Source: CAD feature listing. Evaluate the final solid. Frame: model axes, mm. A direction names the side the tool comes from. Give positions to 0.01 mm unless a question says otherwise; leave off trailing zeros. Write each loop counter-clockwise with the first axis right and the second up, starting at its lowest first coordinate (ties: lowest second). Pieces come first, ordered by that corner, then holes. Notation, with made-up numbers: (49, -2.5) -> (70, -2.5) arc R31 ccw to (70, 32.5) -> close; hole circle Ø8 at (43, -34). An arc over 180 degrees is marked (long way). Write item = value, one per line.
Autodesk Inventor part; units mm, degrees
ref_plane "YZ Plane" through (0, 0, 0) normal (1, 0, 0) x (0, 1, 0)
ref_plane "XZ Plane" through (0, 0, 0) normal (0, 1, 0) x (-1, 0, 0)
ref_plane "XY Plane" through (0, 0, 0) normal (0, 0, 1) x (1, 0, 0)
sketch "Skizze1" plane through (0, 0, 0) normal (0, 0, 1) x (1, 0, 0)
  line L0 (-60, 110) -> (60, 110)
  line L1 (60, 110) -> (60, -10)
  line L2 (60, -10) -> (-60, -10)
  line L3 (-60, -10) -> (-60, 110)
  point P0 (0, 0)
  point P1 (0, 110)
  dimension "d0" = 120
  dimension "d1" = 120
  dimension "d2" = 10
extrude "Extrusion1" add sketch "Skizze1" against normal blind 5
sketch "Skizze2" plane through (0, 0, 0) normal (0, 0, 1) x (1, 0, 0)
  line L0 (-60, -10) -> (-60, 110)
  line L1 (-60, 0) -> (-10.5, 0)
  line L2 (-10.5, 0) -> (-10.5, 110)
  line L3 (-60, 110) -> (60, 110)
  line L4 (-5, 110) -> (-5, 0)
  line L5 (-5, 0) -> (60, 0)
  line L6 (-60, -10) -> (60, -10)
  line L7 (60, -10) -> (-60, -10)
  line L8 (60, 110) -> (60, -10)
  line L9 (-10.5, 110) -> (-5, 110)
  line L10 (-60, -10) -> (60, -10)
  line L11 (-60, 0) -> (-60, -3)
  line L12 (-60, -3) -> (-56, -3)
  line L13 (-56, -3) -> (-56, -7)
  line L14 (-56, -7) -> (-60, -7)
  line L15 (-60, -7) -> (-60, -10)
  line L16 (60, -10) -> (60, -7)
  line L17 (60, -7) -> (56, -7)
  line L18 (56, -7) -> (56, -3)
  line L19 (56, -3) -> (60, -3)
  line L20 (60, 0) -> (60, -3)
  point P0 (0, 0)
  dimension "d6" = 5.5
  dimension "d7" = 10
  dimension "d12" = 4
  dimension "d13" = 3
  dimension "d14" = 3
  dimension "d15" = 4
  dimension "d31" = 65
extrude "Extrusion2" add sketch "Skizze2" along normal blind 180 contours L0 L14 L13 L12 L1 L2 L3 L4 L5 L8 L19 L18 L17 L6
sketch "Skizze3" plane through (-5, 0, 0) normal (1, 0, 0) x (0, 0, -1)
  line L0 (-131, 85) -> (-15, 85) construction
  line L1 (-15, 85) -> (-15, 20) construction
  line L2 (-15, 20) -> (-131, 20) construction
  line L3 (-131, 20) -> (-131, 85) construction
  line L4 (0, 0) -> (0, 110)
  line L5 (0, 0) -> (-180, 0)
  line L6 (-107, 72) -> (-20, 72) construction
  line L7 (-20, 72) -> (-20, 30) construction
  line L8 (-20, 30) -> (-107, 30) construction
  line L9 (-107, 30) -> (-107, 72) construction
  line L10 (-147, 71) -> (-127, 71) construction
  line L11 (-127, 71) -> (-127, 31) construction
  line L12 (-127, 31) -> (-147, 31) construction
  line L13 (-147, 31) -> (-147, 71) construction
  dimension "d16" = 116
  dimension "d17" = 65
  dimension "d18" = 15
  dimension "d19" = 20
  dimension "d27" = 87
  dimension "d28" = 42
  dimension "d29" = 5
  dimension "d30" = 10
  dimension "d32" = 20
  dimension "d33" = 40
  dimension "d34" = 20
  dimension "d35" = 11
hole "Bohrung1" at (-5, 85, 131) at (-5, 20, 131) at (-5, 20, 15) at (-5, 85, 15) at (-5, 72, 107) at (-5, 30, 107) at (-5, 30, 20) at (-5, 72, 20) at (-5, 71, 147) at (-5, 31, 127) direction (-1, 0, 0) diameter 3 end through all
sketch "Skizze4" plane through (-5, 0, 0) normal (1, 0, 0) x (0, 0, -1)
  line L0 (0, 110) -> (-180, 110)
  line L1 (-156.6453, 110) -> (-156.6453, 0)
  line L2 (0, 0) -> (-180, 0)
  line L3 (-156.6453, 0) -> (-180, 0)
  line L4 (-180, 0) -> (-180, 110)
  line L5 (0, -3) -> (-180, -3)
  line L6 (-180, 110) -> (-156.6453, 110)
extrude "Extrusion3" cut sketch "Skizze4" against normal through all
sketch "Skizze5" plane through (-5, 0, 0) normal (1, 0, 0) x (0, 0, -1)
  point P0 (0, 0)
fillet "Rundung1" radius 20 1 edges at (-7.75, 110, 156.6453)
fillet "Rundung2" radius 1.4 6 edges at (58, -7, 180) (56, -5, 180) (58, -3, 180) (-58, -7, 180) (-56, -5, 180) (-58, -3, 180)
fillet "Rundung3" radius 5 3 edges at (-5, 0, 78.3226) (-10.5, 0, 78.3226) (-7.75, 0, 156.6453)
fillet "Rundung4" radius 5 5 edges at (-3.5355, 1.4645, 0) (-5, 57.5, 0) (-37.75, 0, 0) (-10.5, 57.5, 0) (-11.9645, 1.4645, 0)
equation "\"d13\" = d14"
equation "\"d15\" = d12"
properties part number "netzteil_halter_unten"
(1) Section query C-C (z = 52). Return loops of the section in (x, y).
Values follow:
outline = (-60, -10) -> (60, -10) -> (60, -7) -> (56, -7) -> (56, -3) -> (60, -3) -> (60, 0) -> (0, 0) arc R5 cw to (-5, 5) -> (-5, 110) -> (-10.5, 110) -> (-10.5, 5) arc R5 cw to (-15.5, 0) -> (-60, 0) -> (-60, -3) -> (-56, -3) -> (-56, -7) -> (-60, -7) -> close
(2) Pull-direction query (Y, two-part tool) for faces 5 (the face through (56, -5, 88)), 6 (the face through (30, 58, 0)), 7 (the face through (-7.86, 0.94, 158.73)); classes: pulls with the +Y half, pulls with the -Y half, needs draft (parallel to the pull), parting line crosses it, or undercut.
Values follow:
face_5 = undercut
face_6 = needs draft
face_7 = pulls with the +Y half
(3) Section query D-D (y = 98). Return loops of the section in (x, z), plus the area to 3 significant figures.
Values follow:
outline = (-60, -5) -> (60, -5) -> (60, 0) -> (0, 0) arc R5 cw to (-5, 5) -> (-5, 154.98) -> (-10.5, 154.98) -> (-10.5, 5) arc R5 cw to (-15.5, 0) -> (-60, 0) -> close
area = 1,460 mm2
(4) First-contact query: pin 1 (22 mm diameter, centred on x = -33.5, y = 35.5, fed in from +Z); pin 2 (6 mm diameter, centred on x = 15.5, z = 153.5, fed in from +Y); pin 3 (12 mm diameter, centred on y = 53, z = 35.5, fed in from +X). Flat tips, straight axial feed; report the tip coordinate or a pass-through.
Values follow:
pin_1 = 0
pin_2 = 0
pin_3 = -5
(5) Section query A-A (y = 54.5). Return loops of the section in (x, z), plus the area to 3 significant figures.
Values follow:
outline = (-60, -5) -> (60, -5) -> (60, 0) -> (0, 0) arc R5 cw to (-5, 5) -> (-5, 156.65) -> (-10.5, 156.65) -> (-10.5, 5) arc R5 cw to (-15.5, 0) -> (-60, 0) -> close
area = 1,470 mm2
(6) Section query B-B (x = 44.5). Return loops of the section in (y, z), plus the area to 3 significant figures.
Values follow:
outline = (-10, -5) -> (110, -5) -> (110, 0) -> (5, 0) arc R5 cw to (0, 5) -> (0, 180) -> (-10, 180) -> close
area = 2,410 mm2
(7) Material intervals for line 1 (Y direction, x = -9.4, z = 131); line 2 (Y direction, x = -6, z = 107); line 3 (Z direction, x = -8, y = 20), sorted ascending.
Values follow:
line_1 = -10 to 18.5, 21.5 to 83.5, 86.5 to 110
line_2 = -10 to 28.5, 31.5 to 70.5, 73.5 to 110
line_3 = -5 to 13.5, 16.5 to 129.5, 132.5 to 156.65
(8) Access query for faces 1 (the face through (-4, 2, 84)), 2 (the face through (12, 0, 91)), 3 (the face through (-12, 1.43, 84.42)), 4 (the face through (58, -7, 88)). Directions: +Z, -Z, +X, -X, +Y, -Y. A direction counts if a zero-diameter tool reaches every point of the face in a straight line with its end or side. Return the directions, or none.
Values follow:
face_1 = +Z, +X, +Y
face_2 = +Z, +Y
face_3 = +Z, -X, +Y
face_4 = +Z, +X
